Source: CAD feature listing. Evaluate the final solid. Frame: model axes, mm. Give positions to 0.01 mm unless a question says otherwise; leave off trailing zeros. Write each loop counter-clockwise with the first axis right and the second up, starting at its lowest first coordinate (ties: lowest second). Pieces come first, ordered by that corner, then holes.
```python
from build123d import *

# Parameters (mm, degrees)
SKETCH1_W                                         = 78.2
SKETCH1_H                                         = 10
BOSS_EXTRUDE1_DEPTH                               = 10
CSK_FOR_M2_5_FLAT_HEAD_MACHINE_SCREW1_D           = 2.9
CSK_FOR_M2_5_FLAT_HEAD_MACHINE_SCREW1_CSINK_D     = 5.5
CSK_FOR_M2_5_FLAT_HEAD_MACHINE_SCREW1_CSINK_ANGLE = 90
CSK_FOR_M2_5_FLAT_HEAD_MACHINE_SCREW2_D           = 2.9
CSK_FOR_M2_5_FLAT_HEAD_MACHINE_SCREW2_CSINK_D     = 5.5
CSK_FOR_M2_5_FLAT_HEAD_MACHINE_SCREW2_CSINK_ANGLE = 90
CSK_FOR_M2_5_FLAT_HEAD_MACHINE_SCREW3_D           = 2.9
CSK_FOR_M2_5_FLAT_HEAD_MACHINE_SCREW3_CSINK_D     = 5.5
CSK_FOR_M2_5_FLAT_HEAD_MACHINE_SCREW3_CSINK_ANGLE = 90


with BuildPart() as part:
    # Sketch1 → Boss-Extrude1 (new body)
    with BuildSketch(Plane(origin=(0, 0, 0), x_dir=(1, 0, 0), z_dir=(0, 1, 0))):
        with Locations((-39.1, -5)):
            Rectangle(SKETCH1_W, SKETCH1_H)
    extrude(amount=BOSS_EXTRUDE1_DEPTH)

    # CSK for M2.5 Flat Head Machine Screw1 (through all)
    with Locations(Plane.XY.offset(10)):
        with Locations((-5, 5.154214905)):
            CounterSinkHole(CSK_FOR_M2_5_FLAT_HEAD_MACHINE_SCREW1_D / 2, CSK_FOR_M2_5_FLAT_HEAD_MACHINE_SCREW1_CSINK_D / 2, counter_sink_angle=CSK_FOR_M2_5_FLAT_HEAD_MACHINE_SCREW1_CSINK_ANGLE)

    # CSK for M2.5 Flat Head Machine Screw2 (through all)
    with Locations(Plane.XY.offset(10)):
        with Locations((-73.199, 4.414547578)):
            CounterSinkHole(CSK_FOR_M2_5_FLAT_HEAD_MACHINE_SCREW2_D / 2, CSK_FOR_M2_5_FLAT_HEAD_MACHINE_SCREW2_CSINK_D / 2, counter_sink_angle=CSK_FOR_M2_5_FLAT_HEAD_MACHINE_SCREW2_CSINK_ANGLE)

    # CSK for M2.5 Flat Head Machine Screw3 (through all)
    with Locations(Plane(origin=(0, 10, 0), x_dir=(1, 0, 0), z_dir=(0, 1, 0))):
        with Locations((-39.1, -5)):
            CounterSinkHole(CSK_FOR_M2_5_FLAT_HEAD_MACHINE_SCREW3_D / 2, CSK_FOR_M2_5_FLAT_HEAD_MACHINE_SCREW3_CSINK_D / 2, counter_sink_angle=CSK_FOR_M2_5_FLAT_HEAD_MACHINE_SCREW3_CSINK_ANGLE)


solid = part.part
```
1. Section query A-A (z = 5). Return loops of the section in (x, y).
2. Section query B-B (x = -5). Return loops of the section in (y, z).
3. Pin query (flat end, axial travel): P1, Ø4, axis at x = -12.5, z = 3.5, coming from the -Y side. Return the tip coordinate at first contact, or that it passes through.
4. Line query: probe 1 along Z at (x, y) = (-39.1, 2.75); probe 2 along X at (y, z) = (3.25, 5); probe 3 along Y at (x, z) = (-5, 6.5). Output: solid intervals per line, ascending.
5. Pull-direction query (Y, two-part tool) for faces 1 (the flat face through (0, 5, 5)), 2 (the cylindrical face through (-3.55, 5.22, 4.29)), 3 (the flat face through (-40, 10, 2)); classes: pulls with the +Y half, pulls with the -Y half, needs draft (parallel to the pull), parting line crosses it, or undercut.
The answers:
1. outline: (-78.2, 0) - (-40.55, 0) - (-40.55, 8.7) - (-41.85, 10) - (-78.2, 10) - close; (-37.65, 0) - (0, 0) - (0, 10) - (-36.35, 10) - (-37.65, 8.7) - close; hole circle Ø2.9 at (-73.2, 4.41); hole circle Ø2.9 at (-5, 5.15)
2. outline: (0, 0) - (3.7, 0) - (3.7, 8.7) - (2.4, 10) - (0, 10) - close; (6.6, 0) - (10, 0) - (10, 10) - (7.9, 10) - (6.6, 8.7) - close
3. P1: stops at y = 0
4. probe 1: z = 0 to 3.55, 6.45 to 10
4. probe 2: x = -78.2 to -74.06, -72.34 to -40.55, -37.65 to 0
4. probe 3: y = 0 to 3.7, 6.6 to 10
5. face 1: needs draft
5. face 2: undercut
5. face 3: pulls with the +Y half
